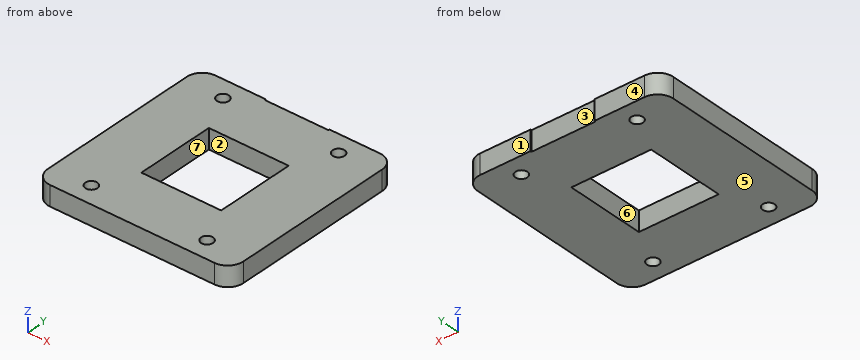
```python
from build123d import *

# Parameters (mm, degrees)
BOSS_EXTRUDE1_DEPTH = 5
SKETCH2_W           = 20
SKETCH2_H           = 20
CUT_EXTRUDE1_DEPTH  = 5
SKETCH5_R           = 1.5
CUT_EXTRUDE2_DEPTH  = 36.007142128
SKETCH6_W           = 16
SKETCH6_H           = 0.8
CUT_EXTRUDE3_DEPTH  = 36.007142128


with BuildPart() as part:
    # Sketch1 → Boss-Extrude1 (new body)
    with BuildSketch(Plane.XY):
        with BuildLine():
            Line((20.59, 24.5), (-20.59, 24.5))
            ThreePointArc((-20.59, 24.5), (-23.354787514, 23.354787514), (-24.5, 20.59))
            Line((-24.5, 20.59), (-24.5, -20.59))
            ThreePointArc((-24.5, -20.59), (-23.354787514, -23.354787514), (-20.59, -24.5))
            Line((-20.59, -24.5), (20.59, -24.5))
            ThreePointArc((20.59, -24.5), (23.354787514, -23.354787514), (24.5, -20.59))
            Line((24.5, -20.59), (24.5, 20.59))
            ThreePointArc((24.5, 20.59), (23.354787514, 23.354787514), (20.59, 24.5))
        make_face()
    extrude(amount=BOSS_EXTRUDE1_DEPTH)

    # Sketch2 → Cut-Extrude1 (cut)
    with BuildSketch(Plane.XY.offset(5)):
        Rectangle(SKETCH2_W, SKETCH2_H)
    extrude(amount=-CUT_EXTRUDE1_DEPTH, mode=Mode.SUBTRACT)

    # Sketch5 → Cut-Extrude2 (cut, through all)
    with BuildSketch(Plane.XY.offset(5)):
        with Locations((-14.5, 19.5)):
            Circle(SKETCH5_R)
        with Locations((14.5, 19.5)):
            Circle(SKETCH5_R)
        with Locations((-14.5, -19.5)):
            Circle(SKETCH5_R)
        with Locations((14.5, -19.5)):
            Circle(SKETCH5_R)
    extrude(amount=-CUT_EXTRUDE2_DEPTH, mode=Mode.SUBTRACT)

    # Sketch6 → Cut-Extrude3 (cut, through all)
    with BuildSketch(Plane(origin=(0, 0, 0), x_dir=(-1, 0, 0), z_dir=(0, 0, -1))):
        with Locations((0, 24.6)):
            Rectangle(SKETCH6_W, SKETCH6_H)
    extrude(amount=-CUT_EXTRUDE3_DEPTH, mode=Mode.SUBTRACT)


solid = part.part
```
Geometry check sheet. Reference: the model listing, model coordinates, mm. Face numbers are marked on the shaded views. A direction names the side the tool comes from. Give positions to 0.01 mm unless a question says otherwise; leave off trailing zeros. Write each loop counter-clockwise with the first axis right and the second up, starting at its lowest first coordinate (ties: lowest second). Pieces come first, ordered by that corner, then holes. Notation, with made-up numbers: (27, 4) -> (73, 4) arc R29 ccw to (73, 31) -> close; hole circle Ø6 at (62.5, -21). An arc over 180 degrees is marked (long way). Use one line per item in the form item = value.
Item 1: Sectioned sample at C-C on y = 19.5. Enter the section's corners in (x, z).
Results list:
outline = (-24.5, 0) -> (-16, 0) -> (-16, 5) -> (-24.5, 5) -> close; (-13, 0) -> (13, 0) -> (13, 5) -> (-13, 5) -> close; (16, 0) -> (24.5, 0) -> (24.5, 5) -> (16, 5) -> close
Item 2: Depth check by flat-ended pin: pin 1 Ø2.5 at (x, y) = (-14.5, -19.5) entering from -Z. Enter the tip coordinate at first touch or a pass-through.
Results list:
pin_1 = through
Item 3: Mould release check, pull along Y, two halves, no side actions. Record for the marked faces 4, 5, 6 and 7: released by +Y, released by -Y, zero draft, split by the parting line, or undercut.
Results list:
face_4 = released by +Y
face_5 = zero draft
face_6 = undercut
face_7 = undercut
Item 4: Scan lines: line 1 (Y direction, x = -14.5, z = 3.65); line 2 (X direction, y = -6.5, z = 1.4); line 3 (Y direction, x = -5, z = 1.8). Record each from-to range of solid material in increasing order.
Results list:
line_1 = -24.5 to -21, -18 to 18, 21 to 24.5
line_2 = -24.5 to -10, 10 to 24.5
line_3 = -24.5 to -10, 10 to 24.2
Item 5: Sectioned sample at B-B on y = 3.5. Enter the section's corners in (x, z).
Results list:
outline = (-24.5, 0) -> (-10, 0) -> (-10, 5) -> (-24.5, 5) -> close; (10, 0) -> (24.5, 0) -> (24.5, 5) -> (10, 5) -> close
Item 6: Access from +Z, -Z, +X, -X, +Y, -Y to the whole of each face (thin tool, end or side, straight path). Record for the marked faces 1, 2 and 3.
Results list:
face_1 = +Z, -Z, +X, -X, +Y
face_2 = +Z, -Z
face_3 = +Z, -Z, +Y
Item 7: Sectioned sample at D-D on z = 3.2. Enter the section's corners in (x, y).
Results list:
outline = (-24.5, -20.59) arc R3.91 ccw to (-20.59, -24.5) -> (20.59, -24.5) arc R3.91 ccw to (24.5, -20.59) -> (24.5, 20.59) arc R3.91 ccw to (20.59, 24.5) -> (8, 24.5) -> (8, 24.2) -> (-8, 24.2) -> (-8, 24.5) -> (-20.59, 24.5) arc R3.91 ccw to (-24.5, 20.59) -> close; hole circle Ø3 at (-14.5, -19.5); hole circle Ø3 at (-14.5, 19.5); hole (-10, -10) -> (10, -10) -> (10, 10) -> (-10, 10) -> close; hole circle Ø3 at (14.5, -19.5); hole circle Ø3 at (14.5, 19.5)
Item 8: Sectioned sample at A-A on x = -6.5. Enter the section's corners in (y, z).
Results list:
outline = (-24.5, 0) -> (-10, 0) -> (-10, 5) -> (-24.5, 5) -> close; (10, 0) -> (24.2, 0) -> (24.2, 5) -> (10, 5) -> close
